Check sheet for the modelled part. Datum: model origin and axes. Units: mm. A direction names the side the tool comes from. Round coordinates to 2 decimals unless told otherwise and drop trailing zeros. Write each loop counter-clockwise with the first axis right and the second up, starting at its lowest first coordinate (ties: lowest second). Pieces come first, ordered by that corner, then holes. Notation, with made-up numbers: M -27,-3 L 8,-3 A22 ccw 8,35 Z; hole C -5.75,86 d1. An arc over 180 degrees is marked long. Answer in a Markdown table with one row per item.
```python
from build123d import *

# Parameters (mm, degrees)
EXTRUDE_1_DEPTH           = 10
HOLE_WIZARD_1_D           = 3.4
HOLE_WIZARD_1_CBORE_D     = 6
HOLE_WIZARD_1_CBORE_DEPTH = 3.4
HOLE_WIZARD_M3_2_D        = 2.5
HOLE_WIZARD_M3_2_DEPTH    = 7.5
HOLE_WIZARD_M3_2_TIP      = 0.751075774


with BuildPart() as part:
    # 草图1 → 凸台-拉伸1 (new body)
    with BuildSketch(Plane(origin=(0, 0, 0), x_dir=(1, 0, 0), z_dir=(0, 1, 0))):
        Polygon((0, 0), (0, 20), (-17, 20), (-17, -20), (0, -20), align=None)
    extrude(amount=EXTRUDE_1_DEPTH)

    # 打孔尺寸(%根据)内六角圆柱头螺钉的类型1 (through all)
    with Locations(Plane(origin=(-4.5, 10, -7.5), x_dir=(0, 0, 1), z_dir=(0, 1, 0))):
        with Locations((0, 0), (15, 0)):
            CounterBoreHole(HOLE_WIZARD_1_D / 2, HOLE_WIZARD_1_CBORE_D / 2, HOLE_WIZARD_1_CBORE_DEPTH)

    # M3 螺纹孔2
    with Locations(Plane(origin=(-17, 5, -12), x_dir=(0, 0, -1), z_dir=(-1, 0, 0))):
        with Locations((0, 0), (-12, 0), (-24, 0)):
            Hole(HOLE_WIZARD_M3_2_D / 2, depth=HOLE_WIZARD_M3_2_DEPTH)
            with Locations((0, 0, -(HOLE_WIZARD_M3_2_DEPTH + HOLE_WIZARD_M3_2_TIP / 2))):  # 118° drill point
                Cone(0, HOLE_WIZARD_M3_2_D / 2, HOLE_WIZARD_M3_2_TIP, mode=Mode.SUBTRACT)


solid = part.part
```
1. Section check D-D, the plane y = 7.5. Record the cut outline in (x, z).
Found:
| item | result |
|---|---|
| outline | M -17,-20 L 0,-20 L 0,20 L -17,20 Z; hole C -4.5,-7.5 d6; hole C -4.5,7.5 d6 |
2. Go/stop test with flat-tipped pins: pin 1 (8 mm diameter, centred on x = -8.5, z = 13.5, fed in from -Y); pin 2 (2 mm diameter, centred on x = -4.5, z = -7.5, fed in from +Y). Record where each tip stops, or that it passes through.
Found:
| item | result |
|---|---|
| pin 1 | stops at y = 0 |
| pin 2 | passes through |
3. Section check A-A, the plane z = 7.5. Record the cut outline in (x, y), and give its area (3 significant figures).
Found:
| item | result |
|---|---|
| outline | M -17,0 L -6.2,0 L -6.2,6.6 L -7.5,6.6 L -7.5,10 L -17,10 Z; M -2.8,0 L 0,0 L 0,10 L -1.5,10 L -1.5,6.6 L -2.8,6.6 Z |
| area | 127 mm2 |
4. Section check C-C, the plane x = -14.25. Record the cut outline in (y, z), and give its area (3 significant figures).
Found:
| item | result |
|---|---|
| outline | M 0,-20 L 10,-20 L 10,20 L 0,20 Z; hole C 5,-12 d2.5; hole C 5,0 d2.5; hole C 5,12 d2.5 |
| area | 385 mm2 |
5. Draft check along X on faces 1 (the face through (-6, 6.6, -6)), 2 (the face through (-8.88, 4.82, -12.12)), 3 (the face through (-6, 6.6, 9)), 4 (the face through (-13.2, 6.22, -0.27)). Enter one of: +X half, -X half, draft (parallel to the pull), parting line (faces both ways), or undercut.
Found:
| item | result |
|---|---|
| face 1 | undercut |
| face 2 | -X half |
| face 3 | undercut |
| face 4 | draft |
6. Section check B-B, the plane x = -4.5. Record the cut outline in (y, z).
Found:
| item | result |
|---|---|
| outline | M 0,-20 L 10,-20 L 10,-10.5 L 6.6,-10.5 L 6.6,-9.2 L 0,-9.2 Z; M 0,-5.8 L 6.6,-5.8 L 6.6,-4.5 L 10,-4.5 L 10,4.5 L 6.6,4.5 L 6.6,5.8 L 0,5.8 Z; M 0,9.2 L 6.6,9.2 L 6.6,10.5 L 10,10.5 L 10,20 L 0,20 Z |
7. Scan lines: L1, parallel to Z at x = -14.5, y = 5; L2, parallel to Y at x = -13.5, z = -12; L3, parallel to X at y = 1, z = 7.5. Record each from-to range of solid material in increasing order.
Found:
| item | result |
|---|---|
| L1 | z = -20 to -13.25, -10.75 to -1.25, 1.25 to 10.75, 13.25 to 20 |
| L2 | y = 0 to 3.75, 6.25 to 10 |
| L3 | x = -17 to -6.2, -2.8 to 0 |
8. Access from +Z, -Z, +X, -X, +Y, -Y to the whole of each face (thin tool, end or side, straight path). Record for faces 5 (the face through (-3.6, 8.32, -4.64)), 6 (the face through (-6.16, 3.25, 7.87)), 7 (the face through (-13.2, 5.76, -12.99)).
Found:
| item | result |
|---|---|
| face 5 | +Y |
| face 6 | +Y, -Y |
| face 7 | -X |
